CAD build for the part. Positions are in the model's coordinates, mm. A direction names the side the tool comes from. Round coordinates to 2 decimals unless told otherwise and drop trailing zeros. Loops run counter-clockwise (first coordinate to the right, second up) from the corner with the lowest first, then second, coordinate; pieces in that order, holes last. Notation, with made-up numbers: (74.5, 29.25) -> (97.5, 29.25) arc R31 ccw to (97.5, 56.25) -> close; hole circle Ø7 at (17, 47.25). An arc over 180 degrees is marked (long way). Answer as CSV lines item,"result".
```python
from build123d import *

# Parameters (mm, degrees)
SKETCH1_R           = 18.5
SKETCH1_R_2         = 11
BOSS_EXTRUDE1_DEPTH = 8
CUT_EXTRUDE1_DEPTH  = 16
SKETCH4_R           = 1
CUT_EXTRUDE2_DEPTH  = 2
CHAMFER1_SIZE       = 0.3


with BuildPart() as part:
    # Sketch1 → Boss-Extrude1 (new body, symmetric)
    with BuildSketch(Plane.XY):
        Circle(SKETCH1_R)
        Circle(SKETCH1_R_2, mode=Mode.SUBTRACT)
    extrude(amount=BOSS_EXTRUDE1_DEPTH, both=True)

    # Sketch3 → Cut-Extrude1 (cut)
    with BuildSketch(Plane(origin=(0, 0, -8), x_dir=(-1, 0, 0), z_dir=(0, 0, -1))):
        with BuildLine():
            Line((-11, -14.874474781), (11, -14.874474781))
            ThreePointArc((11, -14.874474781), (0, -18.5), (-11, -14.874474781))
        make_face()
    extrude(amount=-CUT_EXTRUDE1_DEPTH, mode=Mode.SUBTRACT)

    # Sketch4 → Cut-Extrude2 (cut)
    with BuildSketch(Plane.XZ.offset(14.874474781)):
        Circle(SKETCH4_R)
    extrude(amount=-CUT_EXTRUDE2_DEPTH, mode=Mode.SUBTRACT)

    # Chamfer1
    chamfer1_edges = [part.edges().sort_by_distance(p)[0] for p in [
        (-1, -12.874474781, 0),
    ]]
    chamfer(chamfer1_edges, length=CHAMFER1_SIZE)


solid = part.part
```
Q1. Slice it at B-B, the plane x = 0. Give the cut face in (y, z), and give its area (3 significant figures).
Results:
outline,"(-14.87, -8) -> (-11, -8) -> (-11, 8) -> (-14.87, 8) -> (-14.87, 1) -> (-13.17, 1) -> (-12.87, 0.7) -> (-12.87, -0.7) -> (-13.17, -1) -> (-14.87, -1) -> close; (11, -8) -> (18.5, -8) -> (18.5, 8) -> (11, 8) -> close"
area,"178 mm2"
Q2. Drop flat-ended pins along their axis: pin 1 Ø6 at (x, y) = (5.5, 3) entering from -Z; pin 2 Ø5 at (x, z) = (-12, -1.5) entering from +Y; pin 3 Ø1 at (x, z) = (14.5, -5.5) entering from -Y; pin 4 Ø4 at (y, z) = (10.5, -2.5) entering from -X. Give the stop position or say it passes through.
Results:
pin 1,"through"
pin 2,"y = 15.87"
pin 3,"y = -12.09"
pin 4,"x = -16.43"
Q3. Slice it at D-D, the plane y = -8. Give the cut face in (x, z), and give its area (3 significant figures).
Results:
outline,"(-16.68, -8) -> (-7.55, -8) -> (-7.55, 8) -> (-16.68, 8) -> close; (7.55, -8) -> (16.68, -8) -> (16.68, 8) -> (7.55, 8) -> close"
area,"292 mm2"
Q4. Two-plate mould, pull along Z, no slides. Class faces 1 (the flat face through (0, -14.874, -2)), 2 (the flat face through (8, 9, -8)), 3 (the cylindrical face through (0, -14, -1)): pulls with the +Z half, pulls with the -Z half, needs draft (parallel to the pull), parting line crosses it, or undercut.
Results:
face 1,"needs draft"
face 2,"pulls with the -Z half"
face 3,"undercut"
Q5. Slice it at A-A, the plane y = 0. Give the cut face in (x, z).
Results:
outline,"(-18.5, -8) -> (-11, -8) -> (-11, 8) -> (-18.5, 8) -> close; (11, -8) -> (18.5, -8) -> (18.5, 8) -> (11, 8) -> close"
Q6. Probe L1, parallel to Y at x = -0.5, z = 3; L2, parallel to Z at x = 0, y = -13.75; L3, parallel to Y at x = 0, z = 0.25. List the from-to ranges inside material, lowest first. Write a range as [from, to].
Results:
L1,"[-14.87, -10.99], [10.99, 18.49]"
L2,"[-8, -1], [1, 8]"
L3,"[-12.87, -11], [11, 18.5]"
Q7. Slice it at C-C, the plane z = 0. Give the cut face in (x, y).
Results:
outline,"(-11, -14.87) -> (-1, -14.87) -> (-1, -13.17) -> (-0.7, -12.87) -> (0.7, -12.87) -> (1, -13.17) -> (1, -14.87) -> (11, -14.87) arc R18.5 ccw (long way) to start; hole circle Ø22 at (0, 0)"
Q8. Tool access for faces 4 (the flat face through (0, -12.874, 0)), 5 (the cylindrical face through (0.65, 18.49, 0.11)): list every direction of +Z, -Z, +X, -X, +Y, -Y with a clear straight run to the whole face (end or side of a thin tool).
Results:
face 4,"-Y"
face 5,"+Z, -Z"
